Could you check a few things on this model? Use its own coordinates, in mm. A direction names the side the tool comes from. Round coordinates to 2 decimals unless told otherwise and drop trailing zeros. Order: outer loops, then holes, each group sorted by start corner. A loop starts at its lowest first (then second) coordinate and runs counter-clockwise, first axis right, second up.
```python
from build123d import *

# Parameters (mm, degrees)
EXTRUDE_1_DEPTH    = 13
M2X0_41_AT_2_COUNT = 2
M2X0_41_AT_2_PITCH = 5
M2X0_41_AT_3_COUNT = 2
M2X0_41_AT_3_PITCH = 9.433981132
M2X0_41_AT_4_COUNT = 2
M2X0_41_AT_4_PITCH = 8


with BuildPart() as part:
    # Эскиз1 → Бобышка-Вытянуть1 (new body)
    with BuildSketch(Plane.XY):
        Polygon((-4, 5), (-0.6, 5), (-0.6, 1), (0.6, 1), (0.6, 5), (4, 5), (4, 0), (-4, 0), align=None)
    extrude(amount=EXTRUDE_1_DEPTH)

    # Эскиз2 → Отверстие обработанное метчиком M2x0.41 (revolve, cut)
    with BuildSketch(Plane(origin=(-2.5, 0, 10.5), x_dir=(0, 0, -1), z_dir=(1, 0, 0))):
        Polygon((0, 0), (0, 5), (1.1, 5), (0.8, 4.789937739), (0.8, 0.3), (1.1, 0), align=None)
    m2x0_41 = revolve(axis=Axis((-2.5, -6.35, 10.5), (0, 1, 0)), mode=Mode.SUBTRACT)

    # Отверстие обработанное метчиком M2x0.41 at 2: Отверстие обработанное метчиком M2x0.41 ×2
    with Locations(*[(i * M2X0_41_AT_2_PITCH, 0, 0) for i in range(1, M2X0_41_AT_2_COUNT)]):
        add(m2x0_41, mode=Mode.SUBTRACT)

    # Отверстие обработанное метчиком M2x0.41 at 3: Отверстие обработанное метчиком M2x0.41 ×2
    with Locations(*[Vector(0.52999894, 0, -0.847998304) * (i * M2X0_41_AT_3_PITCH) for i in range(1, M2X0_41_AT_3_COUNT)]):
        add(m2x0_41, mode=Mode.SUBTRACT)

    # Отверстие обработанное метчиком M2x0.41 at 4: Отверстие обработанное метчиком M2x0.41 ×2
    with Locations(*[(0, 0, -i * M2X0_41_AT_4_PITCH) for i in range(1, M2X0_41_AT_4_COUNT)]):
        add(m2x0_41, mode=Mode.SUBTRACT)


solid = part.part
```
Q1. We'd pull the mould along X, two halves only. Please class faces 3 (the flat face through (0.6, 3, 6)), 4 (the flat face through (4, 3, 6)), 5 (the cylindrical face through (-1.72, 2.51, 10.67)), 6 (the flat face through (-4, 2, 6)): released by +X, released by -X, zero draft, split by the parting line, or undercut.
Q2. For faces 1 (the flat face through (0, 1, 6)), 2 (the flat face through (0, 0, 6)), which set-ups out of +Z, -Z, +X, -X, +Y, -Y let a thin tool reach every point of the face, with its end or its side?
Q3. Imagine slicing it at D-D, the plane x = 3. State how many separate pieces and enclosed holes the cut face has, then the cut area to 3 significant figures.
Q4. Imagine slicing it at C-C, the plane z = 10.5. Please give me the cut outline in (x, y), then the cut area to 3 significant figures.
Q5. I need wall thicknesses on L1, parallel to Z at x = 2.5, y = 2.8; L2, parallel to X at y = 1.6, z = 10.5; L3, parallel to X at y = 2.55, z = 10. Which ranges of each line are inside material? Lowest first, please.
Q6. For P1, Ø2, axis at x = 2.5, z = 10.5, coming from the +Y side, with a flat end and sliding along its axis, tell me the tip position at first contact or that it passes through.
Q7. Imagine slicing it at A-A, the plane y = 2.55. Please give me the cut outline in (x, z).
Q8. Imagine slicing it at B-B, the plane x = -2.5. Please give me the cut outline in (y, z), then the cut area to 3 significant figures.
Filled in:
1. face 3: undercut
1. face 4: released by +X
1. face 5: undercut
1. face 6: released by -X
2. face 1: +Z, -Z, +Y
2. face 2: +Z, -Z, +X, -X, -Y
3. separate pieces: 3
3. enclosed holes: 0
3. area: 52.1 mm2
4. outline: (-4, 0) - (-3.6, 0) - (-3.3, 0.3) - (-3.3, 4.79) - (-3.6, 5) - (-4, 5) - close; (-1.7, 0.3) - (-1.4, 0) - (1.4, 0) - (1.7, 0.3) - (1.7, 4.79) - (1.4, 5) - (0.6, 5) - (0.6, 1) - (-0.6, 1) - (-0.6, 5) - (-1.4, 5) - (-1.7, 4.79) - close; (3.3, 0.3) - (3.6, 0) - (4, 0) - (4, 5) - (3.6, 5) - (3.3, 4.79) - close
4. area: 18.9 mm2
5. L1: z = 0 to 1.7, 3.3 to 9.7, 11.3 to 13
5. L2: x = -4 to -3.3, -1.7 to -0.6, 0.6 to 1.7, 3.3 to 4
5. L3: x = -4 to -3.12, -1.88 to -0.6, 0.6 to 1.88, 3.12 to 4
6. P1: stops at y = 4.93
7. outline: (-4, 0) - (-0.6, 0) - (-0.6, 13) - (-4, 13) - close; (0.6, 0) - (4, 0) - (4, 13) - (0.6, 13) - close; hole circle Ø1.6 at (-2.5, 2.5); hole circle Ø1.6 at (-2.5, 10.5); hole circle Ø1.6 at (2.5, 2.5); hole circle Ø1.6 at (2.5, 10.5)
8. outline: (0, 0) - (5, 0) - (5, 1.4) - (4.79, 1.7) - (0.3, 1.7) - (0, 1.4) - close; (0, 3.6) - (0.3, 3.3) - (4.79, 3.3) - (5, 3.6) - (5, 9.4) - (4.79, 9.7) - (0.3, 9.7) - (0, 9.4) - close; (0, 11.6) - (0.3, 11.3) - (4.79, 11.3) - (5, 11.6) - (5, 13) - (0, 13) - close
8. area: 48.7 mm2
